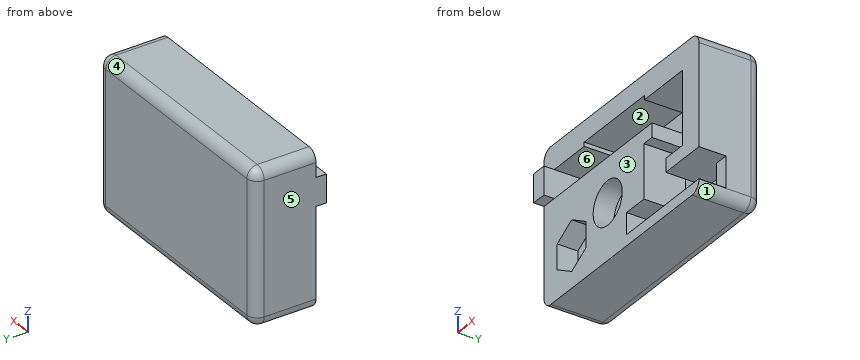
```python
from build123d import *

# Parameters (mm, degrees)
F0_W      = 56
F0_H      = 37
F1_DEPTH  = 15
F3_DEPTH  = 10
F4_W      = 3.7
F4_H      = 6.8
F5_DEPTH  = 2.5
F7_DEPTH  = 5
F8_W      = 3.5
F8_H      = 7.5
F9_DEPTH  = 3.5
F10_R     = 2.5
F11_R     = 5.25
F12_DEPTH = 5


with BuildPart() as f1:
    # F0 (on Front) → F1 (new body)
    with BuildSketch(Plane.XZ):
        Rectangle(F0_W, F0_H)
    extrude(amount=-F1_DEPTH)

    # F2 (on face) → F3 (cut)
    with BuildSketch(Plane.XZ):
        Polygon((-13.468998, 12.5), (-24.3, 12.5), (-24.3, 5.7), (11, 5.7), (11, 2.3), (8.1, 2.3), (8.1, -10.7), (1.8, -10.7), (1.8, -15.9), (28, -15.9), (28, -8.4), (16, -8.4), (16, -5.1), (22, -5.1), (22, 12.5), (8.290843, 12.5), (8.290843, 13.5), (-9.038461, 13.5), (-13.468998, 13.5), align=None)
    extrude(amount=-F3_DEPTH, mode=Mode.SUBTRACT)

    # F4 (on face) → F5 (join)
    with BuildSketch(Plane.XZ):
        with Locations((-26.15, 9.1)):
            Rectangle(F4_W, F4_H)
    extrude(amount=F5_DEPTH)

    # F6 (on face) → F7 (cut)
    with BuildSketch(Plane.XZ):
        Polygon((-23.25, -5.468911), (-23.25, -11.531089), (-18, -14.562178), (-12.75, -11.531089), (-12.75, -5.468911), (-18, -2.437822), align=None)
    extrude(amount=-F7_DEPTH, mode=Mode.SUBTRACT)

    # F8 (on face) → F9 (join)
    with BuildSketch(Plane.XZ.offset(-10)):
        with Locations((26.25, -12.15)):
            Rectangle(F8_W, F8_H)
    extrude(amount=F9_DEPTH)

    # F10
    f10_edges = [f1.edges().sort_by_distance(p)[0] for p in [
        (28, 7.5, -18.5),
        (28, 7.5, 18.5),
        (-28, 7.5, 18.5),
        (-28, 7.5, -18.5),
        (28, 15, 0),
        (0, 15, 18.5),
        (0, 15, -18.5),
        (-28, 15, 0),
    ]]
    fillet(f10_edges, radius=F10_R)

    # F11 (on face) → F12 (cut)
    with BuildSketch(Plane.XZ):
        with Locations((-5, -5)):
            Circle(F11_R)
    extrude(amount=-F12_DEPTH, mode=Mode.SUBTRACT)


solid = f1.part
```
Input: part model. Units: mm. Frame: model coordinates. Face numbers are marked on the shaded views. A direction names the side the tool comes from. Round coordinates to 2 decimals unless told otherwise and drop trailing zeros. Loops run counter-clockwise (first coordinate to the right, second up) from the corner with the lowest first, then second, coordinate; pieces in that order, holes last. Notation, with made-up numbers: (47, -34) - (95, -34) arc R14 cw to (95, -12) - close; hole circle Ø4 at (1.5, 82.25). An arc over 180 degrees is marked (long way). One line per item, written item: value. Start each with the question number.
(1) Section B-B, the plane x = 13. Return loops of the section in (y, z), plus the area to 3 significant figures.
(2) Contact query for flat-ended pins moving along their axis: P1, Ø2, axis at x = -27, y = -1.5, coming from the -Z side; P2, Ø1.5, axis at x = 1.5, z = -11, coming from the -Y side. Output: stop coordinate, or through.
(3) Draft query along Z for the marked faces 4, 5 and 6. Return one class per face: +Z half, -Z half, draft (parallel to the pull), parting line (faces both ways), or undercut.
(4) Section C-C, the plane x = -5. Return loops of the section in (y, z).
(5) Section A-A, the plane z = 1. Return loops of the section in (x, y).
(6) Ray query, line 1 (Z direction, x = -5, y = 3.8); line 2 (Z direction, x = -11.5, y = 3.5); line 3 (Z direction, x = -18.5, y = 9.5). Return the intervals inside material, ascending. Write a range as [from, to].
(7) Section D-D, the plane z = 15. Return loops of the section in (x, y).
(8) Access query for the marked faces 1, 2 and 3. Directions: +Z, -Z, +X, -X, +Y, -Y. A direction counts if a zero-diameter tool reaches every point of the face in a straight line with its end or side. Return the directions, or none.
Results below:
1. outline: (0, -18.5) - (12.5, -18.5) arc R2.5 ccw to (15, -16) - (15, 16) arc R2.5 ccw to (12.5, 18.5) - (0, 18.5) - (0, 12.5) - (10, 12.5) - (10, -15.9) - (0, -15.9) - close
1. area: 268 mm^2
2. P1: z = 5.7
2. P2: y = 0
3. face 4: +Z half
3. face 5: draft
3. face 6: undercut
4. outline: (0, -18.5) - (12.5, -18.5) arc R2.5 ccw to (15, -16) - (15, 16) arc R2.5 ccw to (12.5, 18.5) - (0, 18.5) - (0, 13.5) - (10, 13.5) - (10, 5.7) - (0, 5.7) - (0, 0.25) - (5, 0.25) - (5, -10.25) - (0, -10.25) - close
5. outline: (-28, 0) - (8.1, 0) - (8.1, 10) - (22, 10) - (22, 0) - (28, 0) - (28, 12.5) arc R2.5 ccw to (25.5, 15) - (-25.5, 15) arc R2.5 ccw to (-28, 12.5) - close
6. line 1: [-18.5, -10.25], [0.25, 5.7], [13.5, 18.5]
6. line 2: [-18.5, 5.7], [13.5, 18.5]
6. line 3: [-18.5, 5.7], [12.5, 18.5]
7. outline: (-28, 0) - (28, 0) - (28, 12.5) arc R2.5 ccw to (25.5, 15) - (-25.5, 15) arc R2.5 ccw to (-28, 12.5) - close
8. face 1: -Z, +X, +Y, -Y
8. face 2: -Y
8. face 3: -Z, +X, -X, -Y
